Autodesk Inventor part; units mm, degrees
ref_plane "YZ Plane" through (0, 0, 0) normal (1, 0, 0) x (0, 1, 0)
ref_plane "XZ Plane" through (0, 0, 0) normal (0, 1, 0) x (-1, 0, 0)
ref_plane "XY Plane" through (0, 0, 0) normal (0, 0, 1) x (1, 0, 0)
sketch "Sketch1" plane through (0, 0, 0) normal (0, 0, 1) x (1, 0, 0)
  line L0 (-17.2279, 3.4821) -> (-17.2279, 3.7021)
  line L1 (-13.1179, 4.7021) -> (-16.2279, 4.7021)
  arc A0 (-16.2279, 4.7021) -> (-17.2279, 3.7021) centre (-16.2279, 3.7021) ccw
  line L2 (-15.1179, -1.5179) -> (-13.1179, -1.5179)
  line L3 (-15.1179, -1.5179) -> (-15.1179, 3.4821)
  line L4 (-13.1179, -1.5179) -> (-13.1179, 4.7021)
  line L5 (-17.2279, 3.4821) -> (-13.1179, 3.4821)
  point P0 (-17.2279, 4.7021)
  dimension "d0" = 1.22
  dimension "d2" = 1
  dimension "d7" = 2
  dimension "d8" = 3.11
  dimension "d9" = 4.11
  dimension "d10" = 6.22
  dimension "d11" = 5
revolve "Revolution1" add sketch "Sketch1" angle 360 about axis through (-13.1179, -1.5179, 0) along (0, 1, 0)
sketch "Sketch2" plane through (-13.1179, 4.7021, 0) normal (0, 1, 0) x (1, 0, 0)
  circle A0 centre (0, 0) radius 1.145
  dimension "d13" = 2.29
extrude "Extrusion1" cut sketch "Sketch2" against normal blind 10
fillet "Fillet1" radius 0.2 1 edges at (-14.2629, 4.7021, 0)
sketch "Sketch3" plane through (-13.1179, -1.5179, 0) normal (0, -1, 0) x (1, 0, 0)
  circle A0 centre (0, 0) radius 1.6
  dimension "d17" = 3.2
extrude "Extrusion2" cut sketch "Sketch3" against normal blind 5.2
fillet "Fillet2" radius 0.2 1 edges at (-14.7179, -1.5179, 0)
fillet "Fillet3" radius 0.2 1 edges at (-11.1179, -1.5179, 0)
properties part number "Remache POP Abierto con Rotura de Vástago D4" material "Aluminum 7175 T73 0 Hot Formed"
The model under review builds one solid part; all positions refer to its coordinate system, in mm. Coordinates: 2 decimals unless noted, no trailing zeros. Write each loop counter-clockwise with the first axis right and the second up, starting at its lowest first coordinate (ties: lowest second). Pieces come first, ordered by that corner, then holes. Notation, with made-up numbers: (56, 72.25) -> (103, 72.25) arc R21 ccw to (103, 82.25) -> close; hole circle Ø8 at (-28.75, -6.5). An arc over 180 degrees is marked (long way). Answer in a Markdown table with one row per item.
1. Draft analysis for pull direction Z (two halves, no side actions). For faces 1 (the cylindrical face through (-14.965, 1.115, -0.766)), 2 (the flat face through (-14.5, 4.702, -0.6)), 3 (the cylindrical face through (-14.26, 4.1, -0.05)), 4 (the flat face through (-14, 3.682, -1)), state which applies: +Z half, -Z half, draft (parallel to the pull), parting line (faces both ways), or undercut.
Answers below:
| item | result |
|---|---|
| face 1 | parting line |
| face 2 | draft |
| face 3 | undercut |
| face 4 | undercut |
2. We need section C-C, the plane y = 4. State the section outline as (x, z) points (1 decimal).
Answers below:
| item | result |
|---|---|
| outline | circle Ø8.1 at (-13.1, 0); hole circle Ø2.3 at (-13.1, 0) |
3. We need section B-B, the plane y = 1.25. State the section outline as (x, z) points, and give its area (3 significant figures).
Answers below:
| item | result |
|---|---|
| outline | circle Ø4 at (-13.12, 0); hole circle Ø3.2 at (-13.12, 0) |
| area | 4.52 mm^2 |
4. Wall thickness on probe 1 along Y at (x, z) = (-10.75, -1.5); probe 2 along Z at (x, y) = (-12, -0.75); probe 3 along Z at (x, y) = (-14.5, -0.75): over which ranges is each line inside the solid? List them lowest first. Write a range as [from, to].
Answers below:
| item | result |
|---|---|
| probe 1 | y = [3.48, 4.7] |
| probe 2 | z = [-1.66, -1.14], [1.14, 1.66] |
| probe 3 | z = [-1.45, -0.81], [0.81, 1.45] |
5. Clearance check with flat-ended pins moving along their axes: pin 1 Ø1.5 at (x, z) = (-10, 0) entering from -Y; pin 2 Ø2.5 at (x, z) = (-12.5, 0.5) entering from -Y; pin 3 Ø2 at (x, z) = (-13.12, 0) entering from +Y. State where each tip first meets the part, or that it passes through.
Answers below:
| item | result |
|---|---|
| pin 1 | stops at y = 3.48 |
| pin 2 | stops at y = -1.52 |
| pin 3 | passes through |
